Build history of the part. All positions in model axes, mm. A direction names the side the tool comes from. Round coordinates to 2 decimals unless told otherwise and drop trailing zeros. Write each loop counter-clockwise with the first axis right and the second up, starting at its lowest first coordinate (ties: lowest second). Pieces come first, ordered by that corner, then holes.
from build123d import *

# Parameters (mm, degrees)
SKETCH1_R            = 3.5
SKETCH1_R_2          = 1.5
BOSS_EXTRUDE1_DEPTH  = 2.5
FILLET1_R            = 3
FILLET2_R            = 0.15
M3_CLEARANCE_HOLE1_D = 3.2


with BuildPart() as part:
    # Sketch1 → Boss-Extrude1 (new, symmetric)
    # profile 1 of 3: a face of its own
    with BuildSketch(Plane.XY):
        Circle(SKETCH1_R)
        Circle(SKETCH1_R_2, mode=Mode.SUBTRACT)
    # profile 2 of 3: a face of its own
    with BuildSketch(Plane.XY):
        with BuildLine():
            Line((3.16227766, -1.5), (27.83772234, -1.5))
            ThreePointArc((27.83772234, -1.5), (27.5, 0), (27.83772234, 1.5))
            Line((27.83772234, 1.5), (3.16227766, 1.5))
            ThreePointArc((3.16227766, 1.5), (3.414525722, 0.768774411), (3.5, 0))
            ThreePointArc((3.5, 0), (3.414525722, -0.768774411), (3.16227766, -1.5))
        make_face()
    # profile 3 of 3: a face of its own
    with BuildSketch(Plane.XY):
        with Locations((31, 0)):
            Circle(SKETCH1_R)
        with Locations((31, 0)):
            Circle(SKETCH1_R_2, mode=Mode.SUBTRACT)
    extrude(amount=BOSS_EXTRUDE1_DEPTH, both=True)

    # Fillet1
    fillet1_edges = [part.edges().sort_by_distance(p)[0] for p in [
        (27.83772234, 1.5, 0),
        (27.83772234, -1.5, 0),
        (3.16227766, -1.5, 0),
        (3.16227766, 1.5, 0),
    ]]
    fillet(fillet1_edges, radius=FILLET1_R)

    # Fillet2
    fillet2_edges = [part.edges().sort_by_distance(p)[0] for p in [
        (-3.5, 0, -2.5),
        (-3.5, 0, 2.5),
        (-1.5, 0, 2.5),
        (15.5, 1.5, -2.5),
        (15.5, 1.5, 2.5),
        (34.5, 0, -2.5),
        (34.5, 0, 2.5),
        (29.5, 0, 2.5),
        (15.5, -1.5, -2.5),
        (15.5, -1.5, 2.5),
        (3.513718949, 1.740401367, -2.5),
        (3.513718949, 1.740401367, 2.5),
        (27.486281051, 1.740401367, -2.5),
        (27.486281051, 1.740401367, 2.5),
        (3.513718949, -1.740401367, -2.5),
        (3.513718949, -1.740401367, 2.5),
        (27.486281051, -1.740401367, -2.5),
        (27.486281051, -1.740401367, 2.5),
        (29.5, 0, -2.5),
        (-1.5, 0, -2.5),
    ]]
    fillet(fillet2_edges, radius=FILLET2_R)

    # M3 Clearance Hole1 (through all)
    with Locations(Plane(origin=(0, 0, -2.5), x_dir=(-1, 0, 0), z_dir=(0, 0, -1))):
        with Locations((-31, 0), (0, 0)):
            Hole(M3_CLEARANCE_HOLE1_D / 2)


solid = part.part
1) Which spindle directions (+Z, -Z, +X, -X, +Y, -Y) get a long thin tool onto all of the face, cutting with end or side? Do faces 1 (the cylindrical face through (-3.5, 0.1, 0)), 2 (the cylindrical face through (27.502, 1.747, 0.033)), 3 (the cylindrical face through (3.498, -1.747, -0.033)). Say none if no direction does.
Results:
face 1: +Z, -Z
face 2: +Z, -Z, +Y
face 3: +Z, -Z, -Y
2) Slice it at A-A (x = 0). Write the cut outline in (y, z).
Results:
outline: (-3.5, -2.35) arc R0.15 ccw to (-3.35, -2.5) - (-1.65, -2.5) arc R0.15 ccw to (-1.6, -2.49) - (-1.6, 2.49) arc R0.15 ccw to (-1.65, 2.5) - (-3.35, 2.5) arc R0.15 ccw to (-3.5, 2.35) - close; (1.6, -2.49) arc R0.15 ccw to (1.65, -2.5) - (3.35, -2.5) arc R0.15 ccw to (3.5, -2.35) - (3.5, 2.35) arc R0.15 ccw to (3.35, 2.5) - (1.65, 2.5) arc R0.15 ccw to (1.6, 2.49) - close
3) Slice it at C-C (z = 1.55). Write the cut outline in (x, y).
Results:
outline: (2.53, -2.42) arc R3 cw to (4.69, -1.5) - (26.31, -1.5) arc R3 cw to (28.47, -2.42) arc R3.5 ccw (long way) to (28.47, 2.42) arc R3 cw to (26.31, 1.5) - (4.69, 1.5) arc R3 cw to (2.53, 2.42) arc R3.5 ccw (long way) to start; hole circle Ø3.2 at (0, 0); hole circle Ø3.2 at (31, 0)
4) Slice it at D-D (x = 10). Write the cut outline in (y, z), plus the area to 3 significant figures.
Results:
outline: (-1.5, -2.35) arc R0.15 ccw to (-1.35, -2.5) - (1.35, -2.5) arc R0.15 ccw to (1.5, -2.35) - (1.5, 2.35) arc R0.15 ccw to (1.35, 2.5) - (-1.35, 2.5) arc R0.15 ccw to (-1.5, 2.35) - close
area: 15.0 mm2
5) Wall check: L1, parallel to X at y = 0, z = 0.8; L2, parallel to Y at x = 0, z = 0.55; L3, parallel to X at y = -0.5, z = -0.1. Give the ranges that are in metal, low to high.
Results:
L1: x = -3.5 to -1.6, 1.6 to 29.4, 32.6 to 34.5
L2: y = -3.5 to -1.6, 1.6 to 3.5
L3: x = -3.46 to -1.52, 1.52 to 29.48, 32.52 to 34.46
6) Mould opens along Y. For faces 4 (the cylindrical face through (-1.27, -0.97, 0.03)), 5 (the flat face through (16, 1.5, 0)), 6 (the flat face through (15, -1.5, 0)), 7 (the cylindrical face through (29.4, 0.07, 0.03)) say: released by +Y, released by -Y, zero draft, split by the parting line, or undercut.
Results:
face 4: undercut
face 5: released by +Y
face 6: released by -Y
face 7: undercut
7) Pin check, flat tip, straight feed: pin 1 Ø1 at (x, z) = (22.5, 1.5) entering from -Y. Stop position of the tip, or through.
Results:
pin 1: stops at y = -1.5
8) Slice it at B-B (y = 0). Write the cut outline in (x, z), plus the area to 3 significant figures.
Results:
outline: (-3.5, -2.35) arc R0.15 ccw to (-3.35, -2.5) - (-1.65, -2.5) arc R0.15 ccw to (-1.6, -2.49) - (-1.6, 2.49) arc R0.15 ccw to (-1.65, 2.5) - (-3.35, 2.5) arc R0.15 ccw to (-3.5, 2.35) - close; (1.6, -2.49) arc R0.15 ccw to (1.65, -2.5) - (29.35, -2.5) arc R0.15 ccw to (29.4, -2.49) - (29.4, 2.49) arc R0.15 ccw to (29.35, 2.5) - (1.65, 2.5) arc R0.15 ccw to (1.6, 2.49) - close; (32.6, -2.49) arc R0.15 ccw to (32.65, -2.5) - (34.35, -2.5) arc R0.15 ccw to (34.5, -2.35) - (34.5, 2.35) arc R0.15 ccw to (34.35, 2.5) - (32.65, 2.5) arc R0.15 ccw to (32.6, 2.49) - close
area: 158 mm2
